```python
from build123d import *

# Parameters (mm, degrees)
BOSS_EXTRUDE1_DEPTH  = 350
LPATTERN1_COUNT      = 2
LPATTERN1_PITCH      = 492
MIRROR1_COPY_1_DEPTH = 350


with BuildPart() as part:
    # Sweep1: sweep along a path in Sketch1
    with BuildLine(Plane.XY) as sweep1_path:
        Line((-250, -250), (250, -250))
        Line((250, -250), (250, 250))
        Line((250, 250), (-250, 250))
        Line((-250, 250), (-250, -250))
    # Sketch2 → Sweep1 (sweep)
    with BuildSketch(Plane(origin=(0, -250, 0), x_dir=(1, 0, 0), z_dir=(0, 1, 0))):
        Polygon((212.5, 2), (287.5, 2), (287.5, -38), (283.5, -38), (283.5, -2), (216.5, -2), (216.5, -38), (212.5, -38), align=None)
    sweep(path=sweep1_path.line, transition=Transition.RIGHT)

    # Sweep3: sweep along a path in Sketch4
    with BuildLine(Plane.XY) as sweep3_path:
        Line((-137, 212.5), (-137, -212.5))
    # Sketch5 → Sweep3 (sweep)
    with BuildSketch(Plane(origin=(0, -212.5, 0), x_dir=(1, 0, 0), z_dir=(0, 1, 0))):
        Polygon((-174.5, 2), (-99.5, 2), (-99.5, -38), (-103.5, -38), (-103.5, -2), (-170.5, -2), (-170.5, -38), (-174.5, -38), align=None)
    sweep(path=sweep3_path.line)

    # Sweep4: sweep along a path in Sketch6
    with BuildLine(Plane.XY) as sweep4_path:
        Line((212.5, 137), (-99.5, 137))
    # Sketch7 → Sweep4 (sweep)
    with BuildSketch(Plane.ZY.offset(-212.5)):
        Polygon((-2, 99.5), (-2, 174.5), (38, 174.5), (38, 170.5), (2, 170.5), (2, 103.5), (38, 103.5), (38, 99.5), align=None)
    sweep(path=sweep4_path.line)

    # Sketch8 → Boss-Extrude1 (add)
    with BuildSketch(Plane.XY.offset(2)):
        Polygon((-283.5, 283.5), (-208.5, 283.5), (-208.5, 243.5), (-212.5, 243.5), (-212.5, 279.5), (-279.5, 279.5), (-279.5, 243.5), (-283.5, 243.5), align=None)
    boss_extrude1 = extrude(amount=BOSS_EXTRUDE1_DEPTH)

    # LPattern1: Boss-Extrude1 ×2
    with Locations(*[(i * LPATTERN1_PITCH, 0, 0) for i in range(1, LPATTERN1_COUNT)]):
        add(boss_extrude1)

    # Mirror1: Boss-Extrude1 across plane
    add(boss_extrude1.mirror(Plane.ZX))

    # Mirror1 copy 1 sketch → Mirror1 copy 1 (add)
    with BuildSketch(Plane(origin=(492, 0, 2), x_dir=(1, 0, 0), z_dir=(0, 0, 1))):
        Polygon((-283.5, -283.5), (-208.5, -283.5), (-208.5, -243.5), (-212.5, -243.5), (-212.5, -279.5), (-279.5, -279.5), (-279.5, -243.5), (-283.5, -243.5), align=None)
    extrude(amount=MIRROR1_COPY_1_DEPTH)


solid = part.part
```
The listing builds one solid part. Answer for the finished solid, in the listing's coordinates (mm). A direction names the side the tool comes from. Round coordinates to 2 decimals unless told otherwise and drop trailing zeros. Order: outer loops, then holes, each group sorted by start corner. A loop starts at its lowest first (then second) coordinate and runs counter-clockwise, first axis right, second up. Notation, with made-up numbers: (-22.75, -15.5) -> (-5.75, -15.5) arc R32 ccw to (-5.75, 22.5) -> close; hole circle Ø5 at (6, 45.25). An arc over 180 degrees is marked (long way). Answer as CSV lines item,"result". Start each with the question number.
(1) A tool of negligible diameter and unlimited length cuts with its end or side. For faces 1 (the face through (-193, -212.5, 18)), 2 (the face through (-103.5, -3, 20)), from which of +Z, -Z, +X, -X, +Y, -Y can it reach the whole face along a straight path? Write none if from no direction.
(2) The part is cut by section C-C (x = -88). Determine the outline of the cut face in (y, z).
(3) For a pull along X with two mould halves and no side action, classify faces 3 (the face through (-216.5, -3, 20)), 4 (the face through (-240, -280, 352)), 5 (the face through (-283.5, -263, 193)), 6 (the face through (-212.5, -261, 175)) as +X half, -X half, draft (parallel to the pull), parting line (faces both ways), or undercut.
(4) Flat-ended cylindrical pins translate along their axes: pin 1 Ø20 at (y, z) = (-267, 122.5) entering from -X; pin 2 Ø18 at (y, z) = (262, 207) entering from +X; pin 3 Ø2 at (x, z) = (-281.5, 256.5) entering from +Y. Find the tip coordinate at first contact, or state that the pin passes through.
(5) The part is cut by section B-B (z = 140.5). Count the separate pieces of the cut face and the enclosed holes in it, then the cut area to 3 significant figures.
(6) Find the intervals of material crossed by probe 1 along X at (y, z) = (193, 20.5); probe 2 along X at (y, z) = (251, 43.5); probe 3 along Y at (x, z) = (235, 76), in increasing order. Write a range as from..to.
(7) The part is cut by section A-A (y = -114). Determine the outline of the cut face in (x, z), then the cut area to 3 significant figures.
Evaluation:
1,face 1,"+Z, -Z"
1,face 2,"+Z"
2,outline,"(-287.5, -2) -> (-212.5, -2) -> (-212.5, 38) -> (-216.5, 38) -> (-216.5, 2) -> (-283.5, 2) -> (-283.5, 38) -> (-287.5, 38) -> close; (99.5, -2) -> (174.5, -2) -> (174.5, 38) -> (170.5, 38) -> (170.5, 2) -> (103.5, 2) -> (103.5, 38) -> (99.5, 38) -> close; (212.5, -2) -> (287.5, -2) -> (287.5, 38) -> (283.5, 38) -> (283.5, 2) -> (216.5, 2) -> (216.5, 38) -> (212.5, 38) -> close"
3,face 3,"undercut"
3,face 4,"draft"
3,face 5,"-X half"
3,face 6,"undercut"
4,pin 1,"x = -283.5"
4,pin 2,"x = 283.5"
4,pin 3,"y = 283.5"
5,separate pieces,"4"
5,enclosed holes,"0"
5,area,"2,350 mm²"
6,probe 1,"-287.5..-283.5, -216.5..-212.5, -174.5..-170.5, -103.5..-99.5, 212.5..216.5, 283.5..287.5"
6,probe 2,"-283.5..-279.5, -212.5..-208.5, 208.5..212.5, 279.5..283.5"
6,probe 3,"-283.5..-279.5, 279.5..283.5"
7,outline,"(-287.5, -2) -> (-212.5, -2) -> (-212.5, 38) -> (-216.5, 38) -> (-216.5, 2) -> (-283.5, 2) -> (-283.5, 38) -> (-287.5, 38) -> close; (-174.5, -2) -> (-99.5, -2) -> (-99.5, 38) -> (-103.5, 38) -> (-103.5, 2) -> (-170.5, 2) -> (-170.5, 38) -> (-174.5, 38) -> close; (212.5, -2) -> (287.5, -2) -> (287.5, 38) -> (283.5, 38) -> (283.5, 2) -> (216.5, 2) -> (216.5, 38) -> (212.5, 38) -> close"
7,area,"1,760 mm²"
